```python
from build123d import *

# Parameters (mm, degrees)
SKICA1_W                      = 40
SKICA1_H                      = 85
SKICA1_H_2                    = 35
SKICA1_H_3                    = 30
P_IDAT_VYSUNUT_M1_DEPTH       = 3
SKICA3_W                      = 46
SKICA3_H                      = 156
SKICA3_W_2                    = 40
SKICA3_H_2                    = 150
VYSUNOUT_TENKOST_NN_1_DEPTH   = 28
ODEBRAT_VYSUNUT_M2_DEPTH      = 22
ODEBRAT_VYSUNUT_M2_DEPTH_BACK = 17
SKICA4_W                      = 40
SKICA4_H                      = 24
SKICA4_W_2                    = 6.963710183
SKICA4_W_3                    = 3
SKICA5_W                      = 43
SKICA5_H                      = 3
SKICA5_W_2                    = 40
P_IDAT_VYSUNUT_M2_DEPTH       = 25
SKICA6_W                      = 40
SKICA6_H                      = 24
P_IDAT_VYSUNUT_M3_DEPTH       = 3
SKICA7_W                      = 40
SKICA7_H                      = 35
ODEBRAT_VYSUNUT_M3_DEPTH      = 161.881944295
SKICA8_W                      = 44
SKICA8_H                      = 4
ODEBRAT_VYSUNUT_M4_DEPTH      = 40
SKICA13_W                     = 60
SKICA13_H                     = 85
P_IDAT_VYSUNUT_M7_DEPTH       = 3
SKICA14_W                     = 63
SKICA14_H                     = 91
SKICA14_W_2                   = 57
SKICA14_H_2                   = 85
P_IDAT_VYSUNUT_M8_DEPTH       = 28
SKICA15_W                     = 3
SKICA15_H                     = 85
ODEBRAT_VYSUNUT_M6_DEPTH      = 25
SKICA16_W                     = 46
SKICA16_H                     = 3
P_IDAT_VYSUNUT_M9_DEPTH       = 9
SKICA17_W                     = 110
SKICA17_H                     = 3
ODEBRAT_VYSUNUT_M7_DEPTH      = 34
SKICA21_W                     = 3
SKICA21_H                     = 3
P_IDAT_VYSUNUT_M10_DEPTH      = 2
P_IDAT_VYSUNUT_M11_DEPTH      = 2
SKICA23_R                     = 2
ODEBRAT_VYSUNUT_M10_DEPTH     = 5
ODEBRAT_VYSUNUT_M8_DEPTH      = 173.386194343
ODEBRAT_VYSUNUT_M8_DEPTH_BACK = 173.386194343
SKICA19_R                     = 1.5
SKICA24_R                     = 2
SKICA24_R_2                   = 1.910403137
ODEBRAT_VYSUNUT_M11_DEPTH     = 5


with BuildPart() as part:
    # Skica1 → Přidat vysunutím1 (new body)
    with BuildSketch(Plane.XY):
        with Locations((20, 42.5)):
            Rectangle(SKICA1_W, SKICA1_H)
        with Locations((20, 102.5)):
            Rectangle(SKICA1_W, SKICA1_H_2)
        with Locations((20, 135)):
            Rectangle(SKICA1_W, SKICA1_H_3)
    extrude(amount=-P_IDAT_VYSUNUT_M1_DEPTH)

    # Skica3 → Vysunout tenkostěnný1 (add)
    with BuildSketch(Plane(origin=(0, 0, -3), x_dir=(-1, 0, 0), z_dir=(0, 0, -1))):
        with Locations((-20, 75)):
            Rectangle(SKICA3_W, SKICA3_H)
        with Locations((-20, 75)):
            Rectangle(SKICA3_W_2, SKICA3_H_2, mode=Mode.SUBTRACT)
    extrude(amount=-VYSUNOUT_TENKOST_NN_1_DEPTH)

    # Skica4 → Odebrat vysunutím2 (cut, two sides: drawn at the far end of the back side and taken through both)
    with BuildSketch(Plane.XY.offset(-ODEBRAT_VYSUNUT_M2_DEPTH_BACK)):
        with Locations((20, 100)):
            Rectangle(SKICA4_W, SKICA4_H)
        with Locations((-3.481855092, 100)):
            Rectangle(SKICA4_W_2, SKICA4_H)
        with Locations((41.5, 100)):
            Rectangle(SKICA4_W_3, SKICA4_H)
    extrude(amount=ODEBRAT_VYSUNUT_M2_DEPTH + ODEBRAT_VYSUNUT_M2_DEPTH_BACK, mode=Mode.SUBTRACT)

    # Skica5 → Přidat vysunutím2 (add)
    with BuildSketch(Plane.XY):
        with Locations((21.5, 113.5)):
            Rectangle(SKICA5_W, SKICA5_H)
        with Locations((20, 86.5)):
            Rectangle(SKICA5_W_2, SKICA5_H)
    extrude(amount=P_IDAT_VYSUNUT_M2_DEPTH)

    # Skica6 → Přidat vysunutím3 (add)
    with BuildSketch(Plane.XY.offset(25)):
        with Locations((20, 100)):
            Rectangle(SKICA6_W, SKICA6_H)
    extrude(amount=-P_IDAT_VYSUNUT_M3_DEPTH)

    # Skica7 → Odebrat vysunutím3 (cut, through all)
    with BuildSketch(Plane.XY):
        with Locations((20, 132.5)):
            Rectangle(SKICA7_W, SKICA7_H)
    extrude(amount=-ODEBRAT_VYSUNUT_M3_DEPTH, mode=Mode.SUBTRACT)

    # Skica8 → Odebrat vysunutím4 (cut)
    with BuildSketch(Plane(origin=(0, 153, 0), x_dir=(1, 0, 0), z_dir=(0, 1, 0))):
        with Locations((20, -1)):
            Rectangle(SKICA8_W, SKICA8_H)
    extrude(amount=-ODEBRAT_VYSUNUT_M4_DEPTH, mode=Mode.SUBTRACT)

    # Skica13 → Přidat vysunutím7 (add)
    with BuildSketch(Plane(origin=(0, 0, -3), x_dir=(-1, 0, 0), z_dir=(0, 0, -1))):
        with Locations((30, 42.5)):
            Rectangle(SKICA13_W, SKICA13_H)
    extrude(amount=-P_IDAT_VYSUNUT_M7_DEPTH)

    # Skica14 → Přidat vysunutím8 (add)
    with BuildSketch(Plane(origin=(0, 0, -3), x_dir=(-1, 0, 0), z_dir=(0, 0, -1))):
        with Locations((31.5, 42.5)):
            Rectangle(SKICA14_W, SKICA14_H)
        with Locations((31.5, 42.5)):
            Rectangle(SKICA14_W_2, SKICA14_H_2, mode=Mode.SUBTRACT)
    extrude(amount=-P_IDAT_VYSUNUT_M8_DEPTH)

    # Skica15 → Odebrat vysunutím6 (cut)
    with BuildSketch(Plane.XY.offset(25)):
        with Locations((-1.5, 42.5)):
            Rectangle(SKICA15_W, SKICA15_H)
    extrude(amount=-ODEBRAT_VYSUNUT_M6_DEPTH, mode=Mode.SUBTRACT)

    # Skica16 → Přidat vysunutím9 (add)
    with BuildSketch(Plane.XY.offset(25)):
        with Locations((20, 151.5)):
            Rectangle(SKICA16_W, SKICA16_H)
    extrude(amount=P_IDAT_VYSUNUT_M9_DEPTH)

    # Skica17 → Odebrat vysunutím7 (cut)
    with BuildSketch(Plane.XY.offset(34)):
        with Locations((-10, -1.5)):
            Rectangle(SKICA17_W, SKICA17_H)
    extrude(amount=-ODEBRAT_VYSUNUT_M7_DEPTH, mode=Mode.SUBTRACT)

    # Skica21 → Přidat vysunutím10 (add)
    with BuildSketch(Plane.ZY.offset(63)):
        Polygon((25, 0), (25, 88), (-3, 88), (-3, 0), (0, 0), align=None)
        with Locations((-1.5, -1.5)):
            Rectangle(SKICA21_W, SKICA21_H)
    extrude(amount=P_IDAT_VYSUNUT_M10_DEPTH)

    # Skica22 → Přidat vysunutím11 (add)
    with BuildSketch(Plane(origin=(43, 0, 0), x_dir=(0, 0, -1), z_dir=(1, 0, 0))):
        Polygon((-25, 0), (0, 0), (0, -3), (3, -3), (3, 0), (3, 88), (-22, 88), (-22, 112), (3, 112), (3, 153), (-25, 153), (-34, 153), (-34, 150), (-25, 150), (-25, 112), (-25, 88), align=None)
    extrude(amount=P_IDAT_VYSUNUT_M11_DEPTH)

    # Skica23 → Odebrat vysunutím10 (cut)
    with BuildSketch(Plane.XZ):
        with Locations((42.5, 22.5)):
            Circle(SKICA23_R)
        with Locations((42.5, 2.5)):
            Circle(SKICA23_R)
        with Locations((-62.5, 2.5)):
            Circle(SKICA23_R)
        with Locations((-62.5, 22.5)):
            Circle(SKICA23_R)
    extrude(amount=-ODEBRAT_VYSUNUT_M10_DEPTH, mode=Mode.SUBTRACT)

    # Skica19 → Odebrat vysunutím8 (cut, two sides: drawn at the far end of the back side and taken through both)
    with BuildSketch(Plane(origin=(0, 153, 0), x_dir=(1, 0, 0), z_dir=(0, 1, 0)).offset(-ODEBRAT_VYSUNUT_M8_DEPTH_BACK)):
        with Locations(Location((42, -31, 0), (0, 0, 270))):
            Circle(SKICA19_R)
        with Locations(Location((0, -31, 0), (0, 0, 270))):
            Circle(SKICA19_R)
    extrude(amount=ODEBRAT_VYSUNUT_M8_DEPTH + ODEBRAT_VYSUNUT_M8_DEPTH_BACK, mode=Mode.SUBTRACT)

    # Skica24 → Odebrat vysunutím11 (cut)
    with BuildSketch(Plane.XY.offset(25)):
        with Locations((-62.5, 85)):
            Circle(SKICA24_R)
        with Locations((42.5, 85)):
            Circle(SKICA24_R_2)
    extrude(amount=-ODEBRAT_VYSUNUT_M11_DEPTH, mode=Mode.SUBTRACT)


solid = part.part
```
CAD build for the part. Positions are in the model's coordinates, mm. A direction names the side the tool comes from. Coordinates: 2 decimals unless noted, no trailing zeros. Order: outer loops, then holes, each group sorted by start corner. A loop starts at its lowest first (then second) coordinate and runs counter-clockwise, first axis right, second up.
(1) Saw through at A-A, the plane z = 10. Write the cut outline in (x, y).
Solution:
outline: (-65, 0) - (-60, 0) - (-60, 85) - (40, 85) - (40, 0) - (45, 0) - (45, 88) - (-65, 88) - close; (-3, 112) - (45, 112) - (45, 153) - (-3, 153) - close; hole (0, 115) - (40, 115) - (40, 150) - (0, 150) - close
(2) Which spindle directions (+Z, -Z, +X, -X, +Y, -Y) get a long thin tool onto all of the face, cutting with end or side? Do faces 1 (the face through (-60.653, 2.465, 1.734)), 2 (the face through (-63, 85, 20)), 3 (the face through (20, 151, -1)), 4 (the face through (42, 0, 13)). Say none if no direction does.
Solution:
face 1: -Y
face 2: +Z
face 3: +Y
face 4: +Z, +X, -X, -Y
(3) Drill centre lines: L1, parallel to Y at x = 34, z = 5; L2, parallel to Z at x = 42.5, y = 1.35; L3, parallel to X at y = 150.8, z = 31. Where is each one in solid material? Low to high.
Solution:
L1: y = 85 to 88, 112 to 115, 150 to 153
L2: z = -3 to 0.5, 4.5 to 20.5, 24.5 to 25
L3: x = -3 to -1.5, 1.5 to 40.5, 43.5 to 45
(4) Pin check, flat tips, straight feed: pin 1 Ø12 at (x, z) = (-53.5, 26.5) entering from -Y; pin 2 Ø10 at (x, y) = (29.5, 103.5) entering from -Z; pin 3 Ø3 at (x, z) = (-62.5, 22.5) entering from +Y; pin 4 Ø12 at (x, y) = (20, 125.5) entering from -Z. Stop position of each tip, or through.
Solution:
pin 1: stops at y = 85
pin 2: stops at z = 22
pin 3: stops at y = 88
pin 4: passes through
(5) Saw through at D-D, the plane x = -62.5. Write the cut outline in (y, z), and give its area (3 significant figures).
Solution:
outline: (-3, -3) - (88, -3) - (88, 25) - (87, 25) - (87, 20) - (83, 20) - (83, 25) - (0, 25) - (0, 24.5) - (5, 24.5) - (5, 20.5) - (0, 20.5) - (0, 4.5) - (5, 4.5) - (5, 0.5) - (0, 0.5) - (0, 0) - (-3, 0) - close
area: 2,410 mm2
(6) Mould opens along Y. For faces 5 (the face through (-11, 85, 12)), 6 (the face through (41.1, 151.5, 29.8)), 7 (the face through (40, 132, 14)) say: released by +Y, released by -Y, zero draft, split by the parting line, or undercut.
Solution:
face 5: released by -Y
face 6: zero draft
face 7: undercut
(7) Saw through at B-B, the plane x = 30.5. Write the cut outline in (y, z), and give its area (3 significant figures).
Solution:
outline: (-3, -3) - (88, -3) - (88, 22) - (112, 22) - (112, -3) - (115, -3) - (115, -1) - (113, -1) - (113, 3) - (115, 3) - (115, 25) - (85, 25) - (85, 0) - (-3, 0) - close; (150, -3) - (153, -3) - (153, -1) - (150, -1) - close; (150, 3) - (153, 3) - (153, 34) - (150, 34) - close
area: 595 mm2
(8) Saw through at C-C, the plane y = 14.5. Write the cut outline in (x, z).
Solution:
outline: (-65, -3) - (45, -3) - (45, 25) - (40, 25) - (40, 0) - (-60, 0) - (-60, 25) - (-65, 25) - close
